from build123d import *

# Parameters (mm, degrees)
F0_W     = 50
F0_H     = 50
F1_DEPTH = 2
F2_R     = 24
F3_DEPTH = 25
F5_R     = 2
F6_DEPTH = 2.001


with BuildPart() as f1:
    # F0 (on Top) → F1 (new body)
    with BuildSketch(Plane.XY):
        Rectangle(F0_W, F0_H)
    extrude(amount=F1_DEPTH)

    # F2 (on face) → F3 (cut)
    with BuildSketch(Plane(origin=(0, 0, 0), x_dir=(1, 0, 0), z_dir=(0, 0, -1))):
        Circle(F2_R)
    extrude(amount=-F3_DEPTH, mode=Mode.SUBTRACT)

    # F5 (on face) → F6 (cut, through all)
    with BuildSketch(Plane(origin=(0, 0, 0), x_dir=(1, 0, 0), z_dir=(0, 0, -1))):
        with Locations((-20, 20)):
            Circle(F5_R)
        with Locations((20, 20)):
            Circle(F5_R)
        with Locations((20, -20)):
            Circle(F5_R)
        with Locations((-20, -20)):
            Circle(F5_R)
    extrude(amount=-F6_DEPTH, mode=Mode.SUBTRACT)

    # F4 (on Front) → F7 (revolve)
    with BuildSketch(Plane.XZ):
        Polygon((3.125, 38), (24, 2), (25, 2), (4.125, 38), (4.125, 53), (3.125, 53), align=None)
    revolve(axis=Axis((0, 0, 20), (0, 0, 1)))


solid = f1.part
Check sheet for the modelled part. Datum: model origin and axes. Units: mm. A direction names the side the tool comes from. Round coordinates to 2 decimals unless told otherwise and drop trailing zeros. Loops run counter-clockwise (first coordinate to the right, second up) from the corner with the lowest first, then second, coordinate; pieces in that order, holes last. Notation, with made-up numbers: M 51,83.5 L 105,83.5 A15 cw 105,103.5 Z; hole C 21,54 d11. An arc over 180 degrees is marked long. One line per question, with ' | ' between items. Start each with the question number.
Item 1: Section check D-D (z = 18). Record the boundary of the cut face in (x, y).
Item 2: Section check B-B (x = 20). State how many separate pieces and enclosed holes the cut face has, and give its area (3 significant figures).
Item 3: Set-up check for faces 1 (the face through (3.8, -1.6, 45.6)), 2 (the face through (-18, 19, 2)), 3 (the face through (-23.977, -1.055, 0.986)): record each of +Z, -Z, +X, -X, +Y, -Y from which the full face is reachable in a straight line by a thin tool's end or side.
Item 4: Release check for a two-part mould opening along Y. For faces 4 (the face through (20, 18, 1)), 5 (the face through (18, -21, 2)), 6 (the face through (-1.273, 9.694, 28.252)) record: released by +Y, released by -Y, zero draft, split by the parting line, or undercut.
Item 5: Section check A-A (z = 41.5). Record the boundary of the cut face in (x, y) (3 decimals).
Item 6: Gauge pin test, flat ends, axial feed: pin 1 Ø12 at (x, y) = (8.5, -19.5) entering from -Z; pin 2 Ø1.5 at (x, z) = (4.5, 6) entering from +Y; pin 3 Ø7.5 at (x, y) = (18.5, -10) entering from +Z; pin 4 Ø12.5 at (x, y) = (-18, -14) entering from +Z. Record the tip position at first contact, or that the pin passes through.
Item 7: Scan lines: probe 1 along Y at (x, z) = (20, 1.6); probe 2 along Y at (x, z) = (0, 47.5) (3 decimals); probe 3 along Z at (x, y) = (16, 20). Record each from-to range of solid material in increasing order.
Worked out:
1) outline: C 0,0 d31.44; hole C 0,0 d29.44
2) separate pieces: 3 | enclosed holes: 0 | area: 79.7 mm^2
3) face 1: +Z | face 2: +Z, -X, +Y | face 3: -Z
4) face 4: undercut | face 5: zero draft | face 6: split by the parting line
5) outline: C 0,0 d8.25; hole C 0,0 d6.25
6) pin 1: z = 0 | pin 2: y = 22.7 | pin 3: z = 15.31 | pin 4: z = 16.57
7) probe 1: -25 to -22, -18 to -13.27, 13.27 to 18, 22 to 25 | probe 2: -4.125 to -3.125, 3.125 to 4.125 | probe 3: 0 to 2
